```python
from build123d import *

# Parameters (mm, degrees)
SKETCH1_R           = 149.225
BOSS_EXTRUDE1_DEPTH = 3
SKETCH2_R           = 7.62
CUT_EXTRUDE1_DEPTH  = 2.032


with BuildPart() as part:
    # Sketch1 → Boss-Extrude1 (new body)
    with BuildSketch(Plane(origin=(0, 0, 0), x_dir=(1, 0, 0), z_dir=(0, 1, 0))):
        Circle(SKETCH1_R)
    extrude(amount=BOSS_EXTRUDE1_DEPTH)

    # Sketch2 → Cut-Extrude1 (cut)
    with BuildSketch(Plane(origin=(0, 3, 0), x_dir=(1, 0, 0), z_dir=(0, 1, 0))):
        with Locations((0, 137.4902)):
            Circle(SKETCH2_R)
        with Locations((119.070005971, -68.7451)):
            Circle(SKETCH2_R)
        with Locations((-119.070005971, -68.7451)):
            Circle(SKETCH2_R)
    extrude(amount=-CUT_EXTRUDE1_DEPTH, mode=Mode.SUBTRACT)


solid = part.part
```
Work out the finished part from the listing and answer in its coordinate system (mm). A direction names the side the tool comes from. Round coordinates to 2 decimals unless told otherwise and drop trailing zeros. Write each loop counter-clockwise with the first axis right and the second up, starting at its lowest first coordinate (ties: lowest second). Pieces come first, ordered by that corner, then holes. Notation, with made-up numbers: (72, 3.25) - (115, 3.25) arc R19 ccw to (115, 8.25) - close; hole circle Ø6 at (35.25, 21.5). An arc over 180 degrees is marked (long way). Return JSON: item names as keys, results as strings. Group by question number.
Q1. Each of these flat-tipped pins is pushed along its axis until it touches: pin 1 Ø4.5 at (x, z) = (-1, -138) entering from +Y; pin 2 Ø1 at (y, z) = (0.5, 1) entering from -X. Where does it stop, or does it pass through?
Q2. The mould has two halves that part along X. Classify faces 3 (the flat face through (-2, 3, -2)), 4 (the cylindrical face through (-120.06, 2, 61.19)), 5 (the cylindrical face through (-118.42, 1.48, 90.8)): released by +X, released by -X, zero draft, split by the parting line, or undercut.
Q3. For faces 1 (the flat face through (0, 0.968, -138)), 2 (the flat face through (-2, 0, -2)), determine the directions among +Z, -Z, +X, -X, +Y, -Y from which every point of the face is accessible in a straight line to the end or side of a thin tool.
Q4. The part is cut by section A-A on x = 0. Write down the section's boundary in (y, z) (3 decimals).
Q5. The part is cut by section B-B on y = 2.55. Write down the section's boundary in (x, z) (3 decimals), then the cut area to 3 significant figures.
Q6. The part is cut by section D-D on x = -106. Write down the section's boundary in (y, z), then the cut area to 3 significant figures.
Q7. Find the intervals of material crossed by L1, parallel to Z at x = -118, y = 2.15; L2, parallel to Z at x = -122.5, y = 2.5; L3, parallel to X at y = 0.85, z = 126, in increasing order.
Q8. The part is cut by section C-C on z = -71. Write down the section's boundary in (x, y).
Solved:
{
 "1": {"pin 1": "y = 0.97", "pin 2": "x = -149.22"},
 "2": {"face 3": "zero draft", "face 4": "undercut", "face 5": "split by the parting line"},
 "3": {"face 1": "+Y", "face 2": "+Z, -Z, +X, -X, -Y"},
 "4": {"outline": "(0, -149.225) - (3, -149.225) - (3, -145.11) - (0.968, -145.11) - (0.968, -129.87) - (3, -129.87) - (3, 149.225) - (0, 149.225) - close"},
 "5": {"outline": "circle Ø298.45 at (0, 0); hole circle Ø15.24 at (-119.07, 68.745); hole circle Ø15.24 at (0, -137.49); hole circle Ø15.24 at (119.07, 68.745)", "area": "69,400 mm²"},
 "6": {"outline": "(0, -105.03) - (3, -105.03) - (3, 105.03) - (0, 105.03) - close", "area": "630 mm²"},
 "7": {"L1": "-91.35 to 61.2, 76.29 to 91.35", "L2": "-85.22 to 61.94, 75.55 to 85.22", "L3": "-79.95 to 79.95"},
 "8": {"outline": "(-131.25, 0) - (131.25, 0) - (131.25, 3) - (-131.25, 3) - close"}
}
